Check sheet for the modelled part. Datum: model origin and axes. Units: mm. A direction names the side the tool comes from. Give positions to 0.01 mm unless a question says otherwise; leave off trailing zeros. Order: outer loops, then holes, each group sorted by start corner. A loop starts at its lowest first (then second) coordinate and runs counter-clockwise, first axis right, second up. Notation, with made-up numbers: M -31.5,39 L 16.5,39 A25 ccw 16.5,66 Z; hole C 17.5,-20 d2. An arc over 180 degrees is marked long. Return JSON: item names as keys, results as strings. Group by question number.
Autodesk Inventor part; units mm, degrees
ref_plane "YZ Plane" through (0, 0, 0) normal (1, 0, 0) x (0, 1, 0)
ref_plane "XZ Plane" through (0, 0, 0) normal (0, 1, 0) x (-1, 0, 0)
ref_plane "XY Plane" through (0, 0, 0) normal (0, 0, 1) x (1, 0, 0)
sketch "Sketch1" plane through (0, 0, 0) normal (0, 0, 1) x (1, 0, 0)
  line L0 (0, 0) -> (42, 0)
  line L1 (42, 0) -> (42, 22)
  line L2 (42, 22) -> (0, 22)
  line L3 (0, 22) -> (0, 0)
  line L4 (0, 0) -> (-6.5, 0)
  line L5 (-6.5, 0) -> (-6.5, 27)
  line L6 (-6.5, 27) -> (48.5, 27)
  line L7 (48.5, 27) -> (48.5, -5)
  line L8 (48.5, -5) -> (-6.5, -5)
  line L9 (-6.5, -5) -> (-6.5, 0)
  line L10 (-6.5, 27) -> (-21.5, 27)
  line L11 (-21.5, 27) -> (-21.5, -5)
  line L12 (-21.5, -5) -> (-6.5, -5)
  line L13 (48.5, -5) -> (63.5, -5)
  line L14 (63.5, -5) -> (63.5, 27)
  line L15 (63.5, 27) -> (48.5, 27)
  circle A0 centre (-14, 19) radius 3.1
  circle A1 centre (-14, 3) radius 3.1
  line L16 (21, 22) -> (21, 19)
  circle A2 centre (56, 19) radius 3.1
  circle A3 centre (56, 3) radius 3.1
  dimension "d0" = 42
  dimension "d1" = 22
  dimension "d2" = 6.5
  dimension "d3" = 27
  dimension "d4" = 55
  dimension "d5" = 32
  dimension "d11" = 15
  dimension "d12" = 15
  dimension "d13" = 32
  dimension "d16" = 7.5
  dimension "d17" = 7.5
  dimension "d18" = 8
  dimension "d19" = 8
  dimension "d20" = 6.2
  dimension "d21" = 6.2
extrude "Extrusion1" add sketch "Sketch1" along normal blind 30 contours L5 L6 L7 L8 L9
extrude "Extrusion2" add sketch "Sketch1" against normal blind 5 contours L3 L2 L1 L0 | L5 L6 L7 L8 L9
extrude "Extrusion3" add sketch "Sketch1" against normal blind 5 contours L9 L12 L11 L10 L5 | L15 L14 L13 L7
sketch "Sketch2" plane through (48.5, -5, 30) normal (1, 0, 0) x (0, 0, -1)
  line L0 (29.5, 26) -> (19.5, 26)
  line L1 (19.5, 26) -> (19.5, 6)
  line L2 (19.5, 6) -> (29.5, 6)
  line L3 (29.5, 6) -> (29.5, 26)
  point P0 (30, 5)
extrude "Extrusion4" cut sketch "Sketch2" against normal blind 5
equation "\"d2\" = -0.5 * d0 + 0.5 * d4"
equation "\"d21\" = d20"
properties part number "base"
1) Release check for a two-part mould opening along Y. For faces 6 (the face through (58.864, 17.813, -2.465)), 7 (the face through (20, 27, 12)), 8 (the face through (-14, 11, 0)) record: released by +Y, released by -Y, zero draft, split by the parting line, or undercut.
2) Tool access check on faces 1 (the face through (-21.5, 11, -2)), 2 (the face through (46, 1, 6)), 3 (the face through (42, 11, 15)), 4 (the face through (48.5, 11, 18)), 5 (the face through (-11.136, 17.813, -2.465)). Record the directions out of +Z, -Z, +X, -X, +Y, -Y that give a thin tool (end or side, any length) a straight path to the whole face; none if there is none.
3) Material ranges on line 1 along Y through (x, z) = (56, -2); line 2 along Y through (x, z) = (27, 15); line 3 along X through (y, z) = (7, 15.5), recorded low to high.
4) Sectioned sample at A-A on y = 3. Record the boundary of the cut face in (x, z), then the cut area to 3 significant figures.
5) Sectioned sample at D-D on y = 7. Record the boundary of the cut face in (x, z), then the cut area to 3 significant figures.
6) Sectioned sample at C-C on x = 13.5. Record the boundary of the cut face in (y, z).
7) Depth check by flat-ended pin: P1, Ø6.5, axis at y = 16, z = 10, coming from the +X side; P2, Ø2, axis at y = -0.5, z = 2.5, coming from the -X side; P3, Ø10, axis at x = 56, y = 19, coming from the +Z side; P4, Ø11, axis at y = 15, z = 5, coming from the +X side. Enter the tip coordinate at first touch or a pass-through.
8) Sectioned sample at B-B on x = -14. Record the boundary of the cut face in (y, z), then the cut area to 3 significant figures.
Reply:
{
 "1": {"face 6": "undercut", "face 7": "released by +Y", "face 8": "zero draft"},
 "2": {"face 1": "+Z, -Z, -X, +Y, -Y", "face 2": "+X", "face 3": "+Z", "face 4": "+Z, +X, +Y, -Y", "face 5": "+Z, -Z"},
 "3": {"line 1": "-5 to -0.1, 6.1 to 15.9, 22.1 to 27", "line 2": "-5 to 0, 22 to 27", "line 3": "-6.5 to 0, 42 to 48.5"},
 "4": {"outline": "M -21.5,-5 L -17.1,-5 L -17.1,0 L -21.5,0 Z; M -10.9,-5 L 52.9,-5 L 52.9,0 L 48.5,0 L 48.5,0.5 L 43.5,0.5 L 43.5,10.5 L 48.5,10.5 L 48.5,30 L 42,30 L 42,0 L 0,0 L 0,30 L -6.5,30 L -6.5,0 L -10.9,0 Z; M 59.1,-5 L 63.5,-5 L 63.5,0 L 59.1,0 Z", "area": "703 mm^2"},
 "5": {"outline": "M -21.5,-5 L 63.5,-5 L 63.5,0 L 48.5,0 L 48.5,0.5 L 43.5,0.5 L 43.5,10.5 L 48.5,10.5 L 48.5,30 L 42,30 L 42,0 L 0,0 L 0,30 L -6.5,30 L -6.5,0 L -21.5,0 Z", "area": "765 mm^2"},
 "6": {"outline": "M -5,-5 L 27,-5 L 27,30 L 22,30 L 22,0 L 0,0 L 0,30 L -5,30 Z"},
 "7": {"P1": "x = 48.5", "P2": "x = -6.5", "P3": "z = 0", "P4": "x = 63.5"},
 "8": {"outline": "M -5,-5 L -0.1,-5 L -0.1,0 L -5,0 Z; M 6.1,-5 L 15.9,-5 L 15.9,0 L 6.1,0 Z; M 22.1,-5 L 27,-5 L 27,0 L 22.1,0 Z", "area": "98.0 mm^2"}
}
